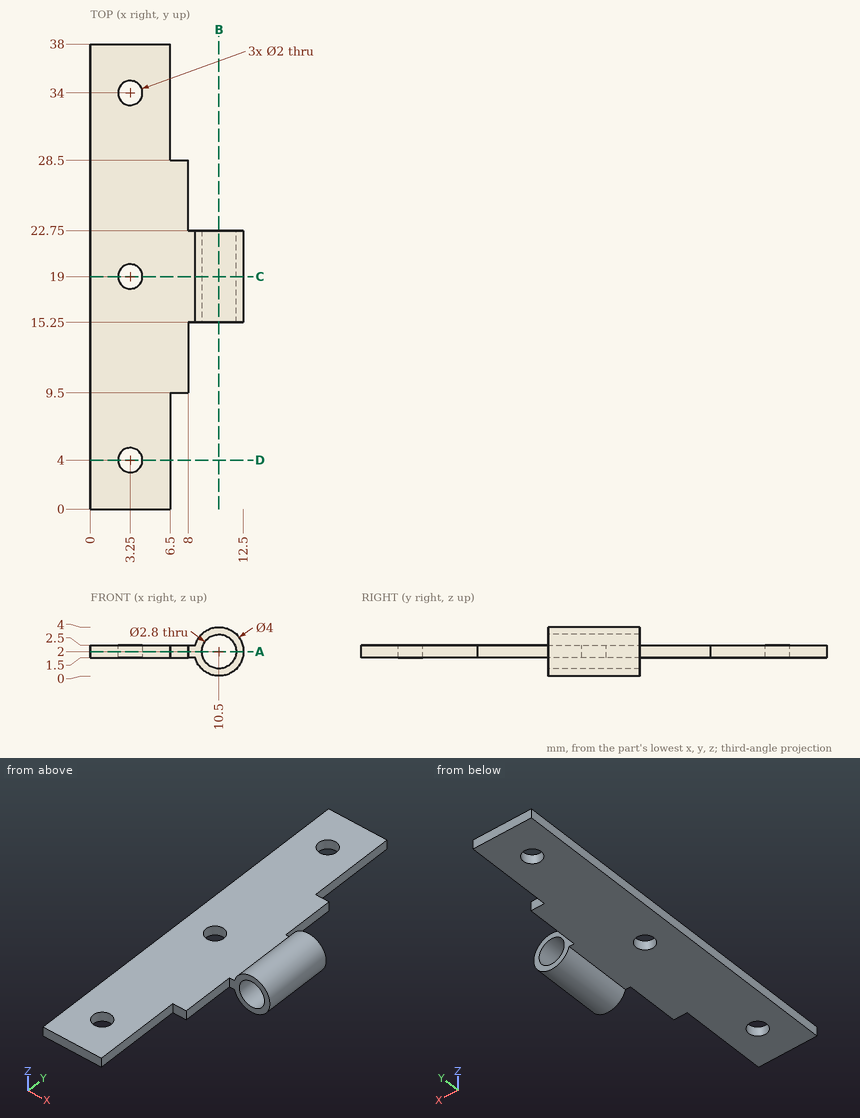
Study the drawing (mm; zero at the part's minimum x, y, z) and answer. Coordinates: 2 decimals unless noted, no trailing zeros. Write each loop counter-clockwise with the first axis right and the second up, starting at its lowest first coordinate (ties: lowest second). Pieces come first, ordered by that corner, then holes.
Q1. Find the intervals of material crossed by line 1 (Y direction, x = 3.25, z = 1.9); line 2 (X direction, y = 34, z = 2.3); line 3 (X direction, y = 19.5, z = 2), in increasing order.
Q2. A cutting plane is placed at B-B, the plane x = 10.5. Give the vertices of the cut face in (y, z).
Q3. A cutting plane is placed at C-C, the plane y = 19. Give the vertices of the cut face in (x, z), then the cut area to 3 significant figures.
Q4. Each of these flat-tipped pins is pushed along its axis until it touches: pin 1 Ø4.5 at (x, y) = (3.5, 25) entering from -Z; pin 2 Ø2 at (x, y) = (7, 13) entering from +Z; pin 3 Ø1.5 at (y, z) = (13, 1.5) entering from +X; pin 4 Ø1 at (x, z) = (11, 2.5) entering from +Y. Where does it stop, or does it pass through?
Q5. A cutting plane is placed at A-A, the plane z = 2. Give the vertices of the cut face in (x, y), then the cut area to 3 significant figures.
Q6. A cutting plane is placed at D-D, the plane y = 4. Give the vertices of the cut face in (x, z).
Findings below:
1. line 1: y = 0 to 3, 5 to 18, 20 to 33, 35 to 38
1. line 2: x = 0 to 2.25, 4.25 to 6.5
1. line 3: x = 0 to 2.38, 4.12 to 9.1, 11.9 to 12.5
2. outline: (15.25, 0) - (22.75, 0) - (22.75, 0.6) - (15.25, 0.6) - close; (15.25, 3.4) - (22.75, 3.4) - (22.75, 4) - (15.25, 4) - close
3. outline: (0, 1.5) - (2.25, 1.5) - (2.25, 2.5) - (0, 2.5) - close; (4.25, 1.5) - (8.56, 1.5) arc R2 ccw (long way) to (8.56, 2.5) - (4.25, 2.5) - close; hole circle Ø2.8 at (10.5, 2)
3. area: 12.9 mm2
4. pin 1: stops at z = 1.5
4. pin 2: stops at z = 2.5
4. pin 3: stops at x = 8
4. pin 4: passes through
5. outline: (0, 0) - (6.5, 0) - (6.5, 9.5) - (8, 9.5) - (8, 15.25) - (9.1, 15.25) - (9.1, 22.75) - (8, 22.75) - (8, 28.5) - (6.5, 28.5) - (6.5, 38) - (0, 38) - close; (11.9, 15.25) - (12.5, 15.25) - (12.5, 22.75) - (11.9, 22.75) - close; hole circle Ø2 at (3.25, 4); hole circle Ø2 at (3.25, 19); hole circle Ø2 at (3.25, 34)
5. area: 279 mm2
6. outline: (0, 1.5) - (2.25, 1.5) - (2.25, 2.5) - (0, 2.5) - close; (4.25, 1.5) - (6.5, 1.5) - (6.5, 2.5) - (4.25, 2.5) - close
